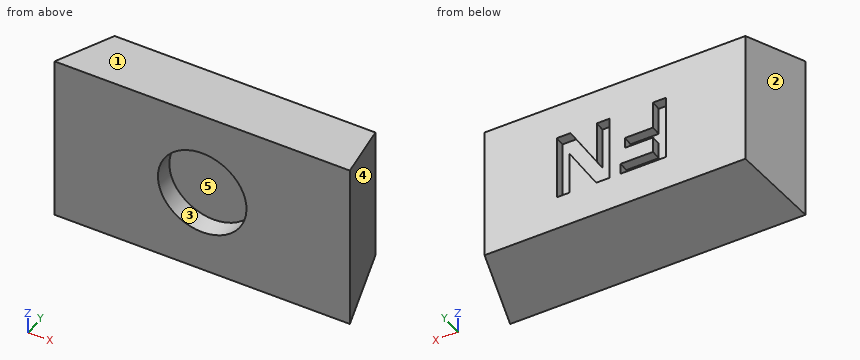
```python
from build123d import *

# Parameters (mm, degrees)
SKETCH1_W               = 12
SKETCH1_H               = 7
BOSS_EXTRUDE1_DEPTH     = 3
CUT_EXTRUDE1_DEPTH      = 7
CUT_EXTRUDE2_DEPTH      = 15.212670404
CUT_EXTRUDE2_DEPTH_BACK = 15.212670404
SKETCH4_R               = 1.8
CUT_EXTRUDE3_DEPTH      = 0.8
CUT_EXTRUDE4_DEPTH      = 0.4


with BuildPart() as part:
    # Sketch1 → Boss-Extrude1 (new body)
    with BuildSketch(Plane(origin=(0, 0, 0), x_dir=(1, 0, 0), z_dir=(0, 1, 0))):
        with Locations((6, 3.5)):
            Rectangle(SKETCH1_W, SKETCH1_H)
    extrude(amount=BOSS_EXTRUDE1_DEPTH)

    # Sketch2 → Cut-Extrude1 (cut)
    with BuildSketch(Plane.XY):
        Polygon((0, 0), (0.7, 3), (0, 3), align=None)
        Polygon((12, 0), (11.3, 3), (12, 3), align=None)
    extrude(amount=-CUT_EXTRUDE1_DEPTH, mode=Mode.SUBTRACT)

    # Sketch3 → Cut-Extrude2 (cut, two sides: drawn at the far end of the back side and taken through both)
    with BuildSketch(Plane(origin=(0, 0, 0), x_dir=(0, 0, -1), z_dir=(1, 0, 0)).offset(-CUT_EXTRUDE2_DEPTH_BACK)):
        Polygon((0, 0), (0.7, 3), (0, 3), align=None)
        Polygon((7, 3), (6.3, 3), (7, 0), align=None)
    extrude(amount=CUT_EXTRUDE2_DEPTH + CUT_EXTRUDE2_DEPTH_BACK, mode=Mode.SUBTRACT)

    # Sketch4 → Cut-Extrude3 (cut)
    with BuildSketch(Plane.XZ):
        with Locations(Location((6, -3.5, 0), (0, 0, 270))):
            Circle(SKETCH4_R)
    extrude(amount=-CUT_EXTRUDE3_DEPTH, mode=Mode.SUBTRACT)

    # Sketch5 → Cut-Extrude4 (cut)
    with BuildSketch(Plane(origin=(0, 3, 0), x_dir=(1, 0, 0), z_dir=(0, 1, 0))):
        Polygon((3.935252413, 2.177234373), (3.935252413, 4.877234373), (5.769867798, 4.877234373), (5.769867798, 4.427234373), (4.454483182, 4.427234373), (4.454483182, 3.769542065), (5.596790874, 3.769542065), (5.596790874, 3.319542065), (4.454483182, 3.319542065), (4.454483182, 2.177234373), align=None)
        Polygon((6.219867798, 2.177234373), (6.219867798, 4.877234373), (6.762355778, 4.877234373), (7.846790874, 3.102114181), (7.846790874, 4.877234373), (8.366021644, 4.877234373), (8.366021644, 2.177234373), (7.806766836, 2.177234373), (6.739098567, 3.924229565), (6.739098567, 2.177234373), align=None)
    extrude(amount=-CUT_EXTRUDE4_DEPTH, mode=Mode.SUBTRACT)


solid = part.part
```
Build history of the part. All positions in model axes, mm. Face numbers are marked on the shaded views. A direction names the side the tool comes from. Round coordinates to 2 decimals unless told otherwise and drop trailing zeros. Write each loop counter-clockwise with the first axis right and the second up, starting at its lowest first coordinate (ties: lowest second). Pieces come first, ordered by that corner, then holes.
1) Band-saw the part on D-D, the plane y = 2.3. List the corners of the cut face in (x, z).
2) Band-saw the part on B-B, the plane z = -4.25. List the corners of the cut face in (x, y).
3) Pin check, flat tips, straight feed: pin 1 (2 mm diameter, centred on x = 6, z = -3.5, fed in from -Y); pin 2 (4 mm diameter, centred on x = 6, z = -4, fed in from -Y); pin 3 (1 mm diameter, centred on y = 1, z = -3.5, fed in from +X). Stop position of each tip, or through.
4) Band-saw the part on C-C, the plane y = 0.2. List the corners of the cut face in (x, z), and give its area (3 significant figures).
5) 3-axis set-ups, long thin cutter, end or side, ignore diameter. For the marked faces 4 and 5: which of +Z, -Z, +X, -X, +Y, -Y reach the whole face in a straight line?
6) Band-saw the part on A-A, the plane x = 6. List the corners of the cut face in (y, z).
7) Mould opens along Z. For the marked faces 1, 2 and 3 say: +Z half, -Z half, draft (parallel to the pull), parting line (faces both ways), or undercut.
8) Drill centre lines: probe 1 along Y at (x, z) = (6.25, -5); probe 2 along X at (y, z) = (0.5, -4); probe 3 along X at (y, z) = (0.4, -3.75). Where is each one in solid material? Low to high.
Ans:
1. outline: (0.54, -6.46) - (11.46, -6.46) - (11.46, -0.54) - (0.54, -0.54) - close
2. outline: (0, 0) - (4.36, 0) - (4.36, 0.8) - (7.64, 0.8) - (7.64, 0) - (12, 0) - (11.3, 3) - (8.37, 3) - (8.37, 2.6) - (7.85, 2.6) - (7.85, 3) - (7.15, 3) - (7.15, 2.6) - (6.22, 2.6) - (6.22, 3) - (4.45, 3) - (4.45, 2.6) - (3.94, 2.6) - (3.94, 3) - (0.7, 3) - close
3. pin 1: stops at y = 0.8
3. pin 2: stops at y = 0
3. pin 3: stops at x = 11.88
4. outline: (0.05, -6.95) - (11.95, -6.95) - (11.95, -0.05) - (0.05, -0.05) - close; hole circle Ø3.6 at (6, -3.5)
4. area: 72.1 mm2
5. face 4: +Z, -Z, +X, +Y
5. face 5: -Y
6. outline: (0, -7) - (3, -6.3) - (3, -0.7) - (0, 0) - (0, -1.7) - (0.8, -1.7) - (0.8, -5.3) - (0, -5.3) - close
7. face 1: +Z half
7. face 2: draft
7. face 3: undercut
8. probe 1: y = 0.8 to 3
8. probe 2: x = 0.12 to 4.27, 7.73 to 11.88
8. probe 3: x = 0.09 to 4.22, 7.78 to 11.91
